Autodesk Inventor part; units mm, degrees
ref_plane "YZ Plane" through (0, 0, 0) normal (1, 0, 0) x (0, 1, 0)
ref_plane "XZ Plane" through (0, 0, 0) normal (0, 1, 0) x (-1, 0, 0)
ref_plane "XY Plane" through (0, 0, 0) normal (0, 0, 1) x (1, 0, 0)
sketch "Sketch1" plane through (0, 0, 0) normal (0, 0, 1) x (1, 0, 0)
  line L0 (0, 0) -> (0, -16) construction
  line L1 (-3.1754, -13.5) -> (-6.3509, -8)
  line L2 (-6.3509, -8) -> (-3.1754, -2.5)
  line L3 (-3.1754, -2.5) -> (3.1754, -2.5)
  line L4 (3.1754, -2.5) -> (6.3509, -8)
  line L5 (6.3509, -8) -> (3.1754, -13.5)
  line L6 (3.1754, -13.5) -> (-3.1754, -13.5)
  point P0 (0, -8)
  point P1 (0, -2.5)
  point P2 (-4.7631, -5.25)
  dimension "d0" = 11
extrude "Extrusion1" add sketch "Sketch1" along normal blind 3.5
hole "Hole1" at (0, -8, 0) direction (0, 0, 1) diameter 6.647 end through all
properties part number "HUDSON-1-89A"
Input: part model. Units: mm. Frame: model coordinates. Round coordinates to 2 decimals unless told otherwise and drop trailing zeros. Order: outer loops, then holes, each group sorted by start corner. A loop starts at its lowest first (then second) coordinate and runs counter-clockwise, first axis right, second up.
1. Cut plane B-B, the plane z = 1.05. Output: boundary loops of the cut face in (x, y), then the cut area to 3 significant figures.
The answers:
outline: (-6.35, -8) - (-3.18, -13.5) - (3.18, -13.5) - (6.35, -8) - (3.18, -2.5) - (-3.18, -2.5) - close; hole circle Ø6.65 at (0, -8)
area: 70.1 mm2
2. Material intervals for line 1 (Y direction, x = 0, z = 1.65); line 2 (X direction, y = -10.75, z = 1.75); line 3 (Y direction, x = 3, z = 0.8), sorted ascending.
The answers:
line 1: y = -13.5 to -11.32, -4.68 to -2.5
line 2: x = -4.76 to -1.87, 1.87 to 4.76
line 3: y = -13.5 to -9.43, -6.57 to -2.5
3. Cut plane A-A, the plane x = 0. Output: boundary loops of the cut face in (y, z), then the cut area to 3 significant figures.
The answers:
outline: (-13.5, 0) - (-11.32, 0) - (-11.32, 3.5) - (-13.5, 3.5) - close; (-4.68, 0) - (-2.5, 0) - (-2.5, 3.5) - (-4.68, 3.5) - close
area: 15.2 mm2
4. Pin query (flat end, axial travel): P1, Ø4, axis at x = -1.5, y = -11, coming from the -Z side; P2, Ø1, axis at y = -4, z = 1, coming from the +X side. Return the tip coordinate at first contact, or that it passes through.
The answers:
P1: stops at z = 0
P2: stops at x = 4.33
5. Cut plane C-C, the plane y = -9. Output: boundary loops of the cut face in (x, z), then the cut area to 3 significant figures.
The answers:
outline: (-5.77, 0) - (-3.17, 0) - (-3.17, 3.5) - (-5.77, 3.5) - close; (3.17, 0) - (5.77, 0) - (5.77, 3.5) - (3.17, 3.5) - close
area: 18.2 mm2
6. Mould query, pull axis Y, two halves, no side actions, for faces 1 (the face through (0, -13.5, 2)), 2 (the face through (3, -10, 0)), 3 (the face through (0, -2.5, 2)), 4 (the face through (-1, -4.83, 1.77)). Classes: released by +Y, released by -Y, zero draft, split by the parting line, or undercut.
The answers:
face 1: released by -Y
face 2: zero draft
face 3: released by +Y
face 4: undercut
7. Cut plane D-D, the plane y = -3.75. Output: boundary loops of the cut face in (x, z).
The answers:
outline: (-3.9, 0) - (3.9, 0) - (3.9, 3.5) - (-3.9, 3.5) - close
